Part model, mm, in its own coordinate system. Round coordinates to 2 decimals unless told otherwise and drop trailing zeros. Write each loop counter-clockwise with the first axis right and the second up, starting at its lowest first coordinate (ties: lowest second). Pieces come first, ordered by that corner, then holes. Notation, with made-up numbers: M 29.5,59 L 60.5,59 A27 ccw 60.5,82 Z; hole C 35.25,31.25 d9. An arc over 180 degrees is marked long. Use a Markdown table: item, result. Add a question column.
1) Drop flat-ended pins along their axis: P1, Ø1, axis at x = -29.5, y = 1.5, coming from the +Z side; P2, Ø1.5, axis at y = -0.5, z = 0.5, coming from the +X side; P3, Ø1.5, axis at y = 0, z = 0.5, coming from the -X side. Give the stop position or say it passes through.
2) Slice it at A-A on y = 0. Write the cut outline in (x, z), plus the area to 3 significant figures.
3) Slice it at C-C on x = 3. Write the cut outline in (y, z), plus the area to 3 significant figures.
4) Wall check: probe 1 along Y at (x, z) = (-33.75, 0); probe 2 along Z at (x, y) = (20, -0.8); probe 3 along X at (y, z) = (0.55, -1). Give the ranges that are in metal, low to high.
```python
from build123d import *

# Parameters (mm, degrees)
SKETCH1_R           = 3
BOSS_EXTRUDE1_DEPTH = 39
SKETCH2_R           = 1.5
CUT_EXTRUDE1_DEPTH  = 7
CUT_EXTRUDE2_START  = -7
SKETCH3_R           = 1.5
CUT_EXTRUDE2_DEPTH  = 7
CHAMFER1_SIZE       = 0.1


with BuildPart() as part:
    # Sketch1 → Boss-Extrude1 (new, symmetric)
    with BuildSketch(Plane(origin=(0, 0, 0), x_dir=(0, 0, -1), z_dir=(1, 0, 0))):
        Circle(SKETCH1_R)
    extrude(amount=BOSS_EXTRUDE1_DEPTH, both=True)

    # Sketch2 → Cut-Extrude1 (cut)
    with BuildSketch(Plane.ZY.offset(39)):
        Circle(SKETCH2_R)
    extrude(amount=-CUT_EXTRUDE1_DEPTH, mode=Mode.SUBTRACT)

    # Sketch3 → Cut-Extrude2 (cut)
    with BuildSketch(Plane(origin=(39, 0, 0), x_dir=(0, 0, -1), z_dir=(1, 0, 0)).offset(CUT_EXTRUDE2_START)):
        with Locations(Location((0, 0, 0), (0, 0, 180))):
            Circle(SKETCH3_R)
    extrude(amount=CUT_EXTRUDE2_DEPTH, mode=Mode.SUBTRACT)

    # Chamfer1
    chamfer1_edges = [part.edges().sort_by_distance(p)[0] for p in [
        (39, 0, -1.5),
        (-39, 0, 3),
        (39, 0, 3),
        (-39, 0, -1.5),
    ]]
    chamfer(chamfer1_edges, length=CHAMFER1_SIZE)


solid = part.part
```
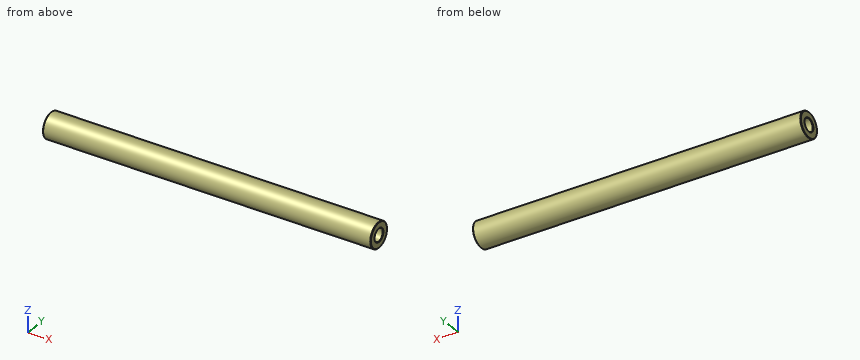
Entries:
| question | item | result |
|---|---|---|
| 1 | P1 | stops at z = 2.83 |
| 1 | P2 | stops at x = 32 |
| 1 | P3 | stops at x = -32 |
| 2 | outline | M -39,-2.9 L -38.9,-3 L 38.9,-3 L 39,-2.9 L 39,-1.6 L 38.9,-1.5 L 32,-1.5 L 32,1.5 L 38.9,1.5 L 39,1.6 L 39,2.9 L 38.9,3 L -38.9,3 L -39,2.9 L -39,1.6 L -38.9,1.5 L -32,1.5 L -32,-1.5 L -38.9,-1.5 L -39,-1.6 Z |
| 2 | area | 426 mm^2 |
| 3 | outline | C 0,0 d6 |
| 3 | area | 28.3 mm^2 |
| 4 | probe 1 | y = -3 to -1.5, 1.5 to 3 |
| 4 | probe 2 | z = -2.89 to 2.89 |
| 4 | probe 3 | x = -32 to 32 |
